```python
from build123d import *

# Parameters (mm, degrees)
AUFSATZ_LINEAR_AUSTRAGEN1_DEPTH = 136
AUFSATZ_LINEAR_AUSTRAGEN2_DEPTH = 2
AUFSATZ_LINEAR_AUSTRAGEN3_DEPTH = 7
SCHNITT_LINEAR_AUSTRAGEN2_DEPTH = 1
SCHNITT_LINEAR_AUSTRAGEN1_REACH = 143.098
SKIZZE14_R                      = 2.5


with BuildPart() as part:
    # Skizze1 → Aufsatz-Linear austragen1 (new body)
    with BuildSketch(Plane.XY):
        with BuildLine():
            Line((7.25, 0), (10.969655115, 0))
            Line((10.969655115, 0), (5.484827557, -9.5))
            Line((5.484827557, -9.5), (-5.484827557, -9.5))
            Line((-5.484827557, -9.5), (-10.969655115, 0))
            Line((-10.969655115, 0), (-7.25, 0))
            ThreePointArc((-7.25, 0), (0, -7.25), (7.25, 0))
        make_face()
    extrude(amount=AUFSATZ_LINEAR_AUSTRAGEN1_DEPTH)

    # Skizze2 → Aufsatz-Linear austragen2 (add)
    with BuildSketch(Plane.XY):
        with BuildLine():
            Line((7.25, 0), (-7.25, 0))
            ThreePointArc((-7.25, 0), (0, -7.25), (7.25, 0))
        make_face()
    extrude(amount=AUFSATZ_LINEAR_AUSTRAGEN2_DEPTH)

    # Skizze3 → Aufsatz-Linear austragen3 (add)
    with BuildSketch(Plane.XY.offset(133)):
        with BuildLine():
            Line((-8.3, 0), (-13.279056191, 0))
            Line((-13.279056191, 0), (-6.639528096, -11.5))
            Line((-6.639528096, -11.5), (6.639528096, -11.5))
            Line((6.639528096, -11.5), (13.279056191, 0))
            Line((13.279056191, 0), (8.3, 0))
            ThreePointArc((8.3, 0), (0, -8.3), (-8.3, 0))
        make_face()
    extrude(amount=AUFSATZ_LINEAR_AUSTRAGEN3_DEPTH)

    # Skizze13 → Schnitt-Linear austragen2 (cut)
    with BuildSketch(Plane(origin=(0, 0, 0), x_dir=(1, 0, 0), z_dir=(0, 1, 0))):
        Polygon((-10.789528096, -140), (10.789528096, -140), (10.789528096, -134.5), (9.169655115, -134.5), (9.169655115, -1), (-9.169655115, -1), (-9.169655115, -134.5), (-10.789528096, -134.5), align=None)
    extrude(amount=-SCHNITT_LINEAR_AUSTRAGEN2_DEPTH, mode=Mode.SUBTRACT)

    # Schnitt-Linear austragen1: up to this face of the body (flat: up to its plane)
    schnitt_linear_austragen1_end = Plane(part.part.faces().sort_by_distance((0, -3.624030572, 2))[0])
    # Skizze14 → Schnitt-Linear austragen1 (cut, up to the picked face)
    with BuildSketch(Plane(origin=(0, 0, 0), x_dir=(-1, 0, 0), z_dir=(0, 0, -1)), mode=Mode.PRIVATE) as schnitt_linear_austragen1_sk1:
        Circle(SKIZZE14_R)
    schnitt_linear_austragen1_tool1 = split(extrude(schnitt_linear_austragen1_sk1.sketch, amount=-SCHNITT_LINEAR_AUSTRAGEN1_REACH, mode=Mode.PRIVATE), bisect_by=schnitt_linear_austragen1_end, keep=Keep.BOTH, mode=Mode.PRIVATE)
    add(schnitt_linear_austragen1_tool1.solids().sort_by(Axis((0, 0, 0), (0, 0, 1)))[0], mode=Mode.SUBTRACT)


solid = part.part
```
Could you check a few things on this model? Use its own coordinates, in mm. A direction names the side the tool comes from. Coordinates: 2 decimals unless noted, no trailing zeros. Order: outer loops, then holes, each group sorted by start corner. A loop starts at its lowest first (then second) coordinate and runs counter-clockwise, first axis right, second up. Notation, with made-up numbers: M -2,19.5 L 20,19.5 A27 ccw 20,51.5 Z; hole C 35,46 d10. An arc over 180 degrees is marked long. Use a Markdown table: item, result. Add a question column.
Q1. I want a section at A-A on x = 0. List the corners of the cut face in (y, z) for me.
Q2. Which directions (+Z, -Z, +X, -X, +Y, -Y) give clear straight access to the entire face, cutting with the end or side of a thin tool? Please do faces 1 (the flat face through (0, -8, 136)), 2 (the flat face through (0, -10, 133)), 3 (the flat face through (0, -9.5, 66)), 4 (the flat face through (8.266, -4.684, 65.569)), 5 (the flat face through (9.913, -5.83, 136.451)).
Q3. I'm going to push flat-ended pins straight in: pin 1 (3.5 mm diameter, centred on x = 2.5, z = 61.5, fed in from -Y); pin 2 (0.5 mm diameter, centred on x = -10, y = -0.5, fed in from +Z); pin 3 (0.8 mm diameter, centred on y = -0.5, z = 138.5, fed in from +X). Where does each tip first touch, or does it pass through?
Q4. We'd pull the mould along X, two halves only. Please class faces 6 (the flat face through (8, -1, 70)), 7 (the flat face through (0, -11.5, 136)), 8 (the flat face through (-8.2, -4.8, 65.6)): pulls with the +X half, pulls with the -X half, needs draft (parallel to the pull), parting line crosses it, or undercut.
Q5. I want a section at B-B on z = 49. List the corners of the cut face in (x, y) for me.
Q6. If I drill on L1, parallel to Z at x = 8.25, y = -7; L2, parallel to X at y = -5.5, z = 91.5; L3, parallel to Z at x = -4.75, y = -2, over which ranges is the centre line in solid material (lowest first)?
Checked values:
| question | item | result |
|---|---|---|
| 1 | outline | M -11.5,133 L -9.5,133 L -9.5,0 L -2.5,0 L -2.5,2 L -7.25,2 L -7.25,136 L -8.3,136 L -8.3,140 L -11.5,140 Z |
| 2 | face 1 | +Z, +Y |
| 2 | face 2 | -Z, -Y |
| 2 | face 3 | -Z, +X, -X, -Y |
| 2 | face 4 | -Z, +X, -Y |
| 2 | face 5 | +Z, -Z, +X, -Y |
| 3 | pin 1 | y = -9.5 |
| 3 | pin 2 | z = 134.5 |
| 3 | pin 3 | x = 13.22 |
| 4 | face 6 | undercut |
| 4 | face 7 | needs draft |
| 4 | face 8 | pulls with the -X half |
| 5 | outline | M -10.97,0 L -5.48,-9.5 L 5.48,-9.5 L 10.97,0 L 9.17,0 L 9.17,-1 L 7.18,-1 A7.25 cw -7.18,-1 L -9.17,-1 L -9.17,0 Z |
| 6 | L1 | 133 to 140 |
| 6 | L2 | -7.79 to -4.72, 4.72 to 7.79 |
| 6 | L3 | 0 to 2 |
